```python
from build123d import *

# Parameters (mm, degrees)
BOSS_EXTRUDE1_DEPTH      = 914.4
BOSS_EXTRUDE1_DEPTH_BACK = 914.4


with BuildPart() as part:
    # Sketch1 → Boss-Extrude1 (new body, two sides)
    with BuildSketch(Plane(origin=(0, 0, 0), x_dir=(0, 0, -1), z_dir=(1, 0, 0))) as boss_extrude1_sk:
        with BuildLine():
            Line((0, 76.2), (0, 0))
            Line((0, 0), (76.2, 0))
            Line((76.2, 0), (76.2, 1.27))
            ThreePointArc((76.2, 1.27), (74.712102448, 4.862102448), (71.12, 6.35))
            Line((71.12, 6.35), (11.43, 6.35))
            ThreePointArc((11.43, 6.35), (7.837897552, 7.837897552), (6.35, 11.43))
            Line((6.35, 11.43), (6.35, 71.12))
            ThreePointArc((6.35, 71.12), (4.862102448, 74.712102448), (1.27, 76.2))
            Line((1.27, 76.2), (0, 76.2))
        make_face()
    extrude(amount=BOSS_EXTRUDE1_DEPTH)
    extrude(boss_extrude1_sk.sketch, amount=-BOSS_EXTRUDE1_DEPTH_BACK)


solid = part.part
```
The listing builds one solid part. Answer for the finished solid, in the listing's coordinates (mm). A direction names the side the tool comes from. Coordinates: 2 decimals unless noted, no trailing zeros. Write each loop counter-clockwise with the first axis right and the second up, starting at its lowest first coordinate (ties: lowest second). Pieces come first, ordered by that corner, then holes. Notation, with made-up numbers: (-3.5, -26) - (31.5, -26) arc R18 cw to (31.5, -20) - close; hole circle Ø2 at (64, 31.25). An arc over 180 degrees is marked (long way). Return JSON: item names as keys, results as strings. Group by question number.
1. Given pin 1 (3 mm diameter, centred on x = 611, y = 14, fed in from -Z); pin 2 (3 mm diameter, centred on x = 18, z = -63.5, fed in from +Y), each flat-ended and moving along its own axis, determine where each tip first touches the part or whether it passes through.
2. Straight lines are drawn through the part: L1, parallel to Y at x = -220.5, z = -70; L2, parallel to Z at x = -427, y = 33; L3, parallel to Y at x = -399, z = -72.5. For each, find the intervals that lie inside material, in ascending order.
3. A cutting plane is placed at B-B, the plane z = -39.5. Determine the outline of the cut face in (x, y).
4. Which of the six approach directions +Z, -Z, +X, -X, +Y, -Y give full straight-line access (tool end or side, diameter ignored) to faces 1 (the flat face through (13, 6.35, -42)), 2 (the flat face through (13, 39, 0))?
5. A cutting plane is placed at C-C, the plane y = 30. Determine the outline of the cut face in (x, z).
6. A cutting plane is placed at A-A, the plane x = -509. Determine the outline of the cut face in (y, z), plus the area to 3 significant figures.
Ans:
{
 "1": {"pin 1": "z = -6.35", "pin 2": "y = 6.35"},
 "2": {"L1": "0 to 6.35", "L2": "-6.35 to 0", "L3": "0 to 6.16"},
 "3": {"outline": "(-914.4, 0) - (914.4, 0) - (914.4, 6.35) - (-914.4, 6.35) - close"},
 "4": {"face 1": "-Z, +X, -X, +Y", "face 2": "+Z, +X, -X, +Y, -Y"},
 "5": {"outline": "(-914.4, -6.35) - (914.4, -6.35) - (914.4, 0) - (-914.4, 0) - close"},
 "6": {"outline": "(0, -76.2) - (1.27, -76.2) arc R5.08 ccw to (6.35, -71.12) - (6.35, -11.43) arc R5.08 cw to (11.43, -6.35) - (71.12, -6.35) arc R5.08 ccw to (76.2, -1.27) - (76.2, 0) - (0, 0) - close", "area": "922 mm²"}
}
